```python
from build123d import *

# Parameters (mm, degrees)
F1_DEPTH = 40
F4_D     = 9
F4_DEPTH = 12
F5_D     = 9
F5_DEPTH = 12
F7_D     = 7
F8_R     = 5


with BuildPart() as f1:
    # F0 (on Front) → F1 (new body, symmetric)
    with BuildSketch(Plane.XZ):
        Polygon((0, 29), (0, 0), (50, 0), (50, 2.5), (2.5, 2.5), (2.5, 26.5), (397.5, 26.5), (397.5, 2.5), (350, 2.5), (350, 0), (400, 0), (400, 29), align=None)
    extrude(amount=F1_DEPTH, both=True)

    # F4
    with Locations(Plane.XY.offset(2.5)):
        with Locations((370, 0)):
            Hole(F4_D / 2, depth=F4_DEPTH)

    # F5
    with Locations(Plane.XY.offset(2.5)):
        with Locations((30, 0)):
            Hole(F5_D / 2, depth=F5_DEPTH)

    # F7 (through all)
    with Locations(Plane.XY.offset(29)):
        with Locations((171, 17), (229, 17), (229, -17), (171, -17)):
            Hole(F7_D / 2)

    # F8
    f8_edges = [f1.edges().sort_by_distance(p)[0] for p in [
        (0, 0, 29),
        (0, 0, 0),
        (400, 0, 29),
        (400, 0, 0),
        (2.5, 0, 2.5),
        (2.5, 0, 26.5),
        (397.5, 0, 2.5),
        (397.5, 0, 26.5),
    ]]
    fillet(f8_edges, radius=F8_R)


solid = f1.part
```
The listing builds one solid part. Answer for the finished solid, in the listing's coordinates (mm). A direction names the side the tool comes from. Give positions to 0.01 mm unless a question says otherwise; leave off trailing zeros. Order: outer loops, then holes, each group sorted by start corner. A loop starts at its lowest first (then second) coordinate and runs counter-clockwise, first axis right, second up. Notation, with made-up numbers: (-30.5, 25) -> (-21.5, 25) arc R17 ccw to (-21.5, 45) -> close; hole circle Ø6 at (35, -32.5). An arc over 180 degrees is marked (long way). Write each question's results on one line, items separated by ' | '.
Q1. Determine the mould class of faces 4 (the face through (365.84, -1.72, 1.23)), 5 (the face through (199, -40, 27)), 6 (the face through (377, -1, 0)), 7 (the face through (167.66, -15.95, 27.73)) for opening direction Y: pulls with the +Y half, pulls with the -Y half, needs draft (parallel to the pull), parting line crosses it, or undercut.
Checked values:
face 4: undercut | face 5: pulls with the -Y half | face 6: needs draft | face 7: undercut
Q2. The part is cut by section B-B, the plane y = 0. Give the vertices of the cut face in (x, z), and give its area (4 significant figures).
Checked values:
outline: (0, 5) arc R5 ccw to (5, 0) -> (25.5, 0) -> (25.5, 2.5) -> (7.5, 2.5) arc R5 cw to (2.5, 7.5) -> (2.5, 21.5) arc R5 cw to (7.5, 26.5) -> (392.5, 26.5) arc R5 cw to (397.5, 21.5) -> (397.5, 7.5) arc R5 cw to (392.5, 2.5) -> (374.5, 2.5) -> (374.5, 0) -> (395, 0) arc R5 ccw to (400, 5) -> (400, 24) arc R5 ccw to (395, 29) -> (5, 29) arc R5 ccw to (0, 24) -> close; (34.5, 0) -> (50, 0) -> (50, 2.5) -> (34.5, 2.5) -> close; (350, 0) -> (365.5, 0) -> (365.5, 2.5) -> (350, 2.5) -> close | area: 1,325 mm^2
Q3. Each of these flat-tipped pins is pushed along its axis until it touches: P1, Ø10.5, axis at x = 30, y = 0, coming from the -Z side; P2, Ø2, axis at y = -23, z = 3, coming from the +X side; P3, Ø2, axis at y = 15, z = 2, coming from the +X side; P4, Ø4, axis at x = 236, y = 8.5, coming from the -Z side. Where does it stop, or does it pass through?
Checked values:
P1: stops at z = 0 | P2: stops at x = 399.9 | P3: stops at x = 399.58 | P4: stops at z = 26.5
Q4. Which of the six approach directions +Z, -Z, +X, -X, +Y, -Y give full straight-line access (tool end or side, diameter ignored) to faces 1 (the face through (25.708, 1.352, 1.232)), 2 (the face through (225.66, -15.95, 27.73)), 3 (the face through (2.5, -1, 14))?
Checked values:
face 1: -Z | face 2: +Z, -Z | face 3: +Y, -Y
Q5. The part is cut by section A-A, the plane z = 13. Give the vertices of the cut face in (x, y), and give its area (3 significant figures).
Checked values:
outline: (0, -40) -> (2.5, -40) -> (2.5, 40) -> (0, 40) -> close; (397.5, -40) -> (400, -40) -> (400, 40) -> (397.5, 40) -> close | area: 400 mm^2
Q6. Straight lines are drawn through the part: probe 1 along Z at (x, y) = (374, 31.5); probe 2 along Y at (x, z) = (229, 28.45); probe 3 along Y at (x, z) = (30, 1.45). For each, find the intervals that lie inside material, in ascending order. Write a range as from..to.
Checked values:
probe 1: z = 0..2.5, 26.5..29 | probe 2: y = -40..-20.5, -13.5..13.5, 20.5..40 | probe 3: y = -40..-4.5, 4.5..40
Q7. The part is cut by section C-C, the plane x = 30. Give the vertices of the cut face in (y, z), and give its area (4 significant figures).
Checked values:
outline: (-40, 0) -> (-4.5, 0) -> (-4.5, 2.5) -> (-40, 2.5) -> close; (-40, 26.5) -> (40, 26.5) -> (40, 29) -> (-40, 29) -> close; (4.5, 0) -> (40, 0) -> (40, 2.5) -> (4.5, 2.5) -> close | area: 377.5 mm^2
Q8. The part is cut by section D-D, the plane x = 171. Give the vertices of the cut face in (y, z), and give its area (3 significant figures).
Checked values:
outline: (-40, 26.5) -> (-20.5, 26.5) -> (-20.5, 29) -> (-40, 29) -> close; (-13.5, 26.5) -> (13.5, 26.5) -> (13.5, 29) -> (-13.5, 29) -> close; (20.5, 26.5) -> (40, 26.5) -> (40, 29) -> (20.5, 29) -> close | area: 165 mm^2
